Design review of the part shown in the three views and the two pictorial views. Dimensions are in mm from the part's minimum x, y and z. Coordinates: 2 decimals unless noted, no trailing zeros. Loops run counter-clockwise (first coordinate to the right, second up) from the corner with the lowest first, then second, coordinate; pieces in that order, holes last. Notation, with made-up numbers: (16, 66.5) -> (74, 66.5) arc R11 cw to (74, 80.5) -> close; hole circle Ø7 at (2.5, 72.25). An arc over 180 degrees is marked (long way). One line per item, written item: value. Start each with the question number.
1. Insertion check: pin 1 (3 mm diameter, centred on x = 2, z = 53, fed in from -Y); pin 2 (1 mm diameter, centred on y = 44, z = 12, fed in from -X); pin 3 (1.5 mm diameter, centred on x = 3, y = 40, fed in from -Z); pin 4 (2.5 mm diameter, centred on x = 3, y = 39, fed in from +Z). Each pin has a flat end and moves straight along its axis. Give the tip position at first contact, or say it passes through.
2. Add section D-D on y = 53. Write out the cut boundary in (x, z), plus the area to 3 significant figures.
3. Add section C-C on x = 2.2. Write out the cut boundary in (y, z).
4. Draft analysis for pull direction Z (two halves, no side actions). For the marked faces 1, 2 and 3, state which applies: pulls with the +Z half, pulls with the -Z half, needs draft (parallel to the pull), parting line crosses it, or undercut.
5. For probe 1 along Y at (x, z) = (4.8, 30.5) (1 decimal); probe 2 along Z at (x, y) = (2.7, 27.5) (1 decimal); probe 3 along Y at (x, z) = (4.3, 32), list the stretches that pass through material, from the lowest coordinate up.
6. Add section B-B on z = 30. Write out the cut boundary in (x, y), plus the area to 3 significant figures.
7. Add section A-A on y = 30. Write out the cut boundary in (x, z).
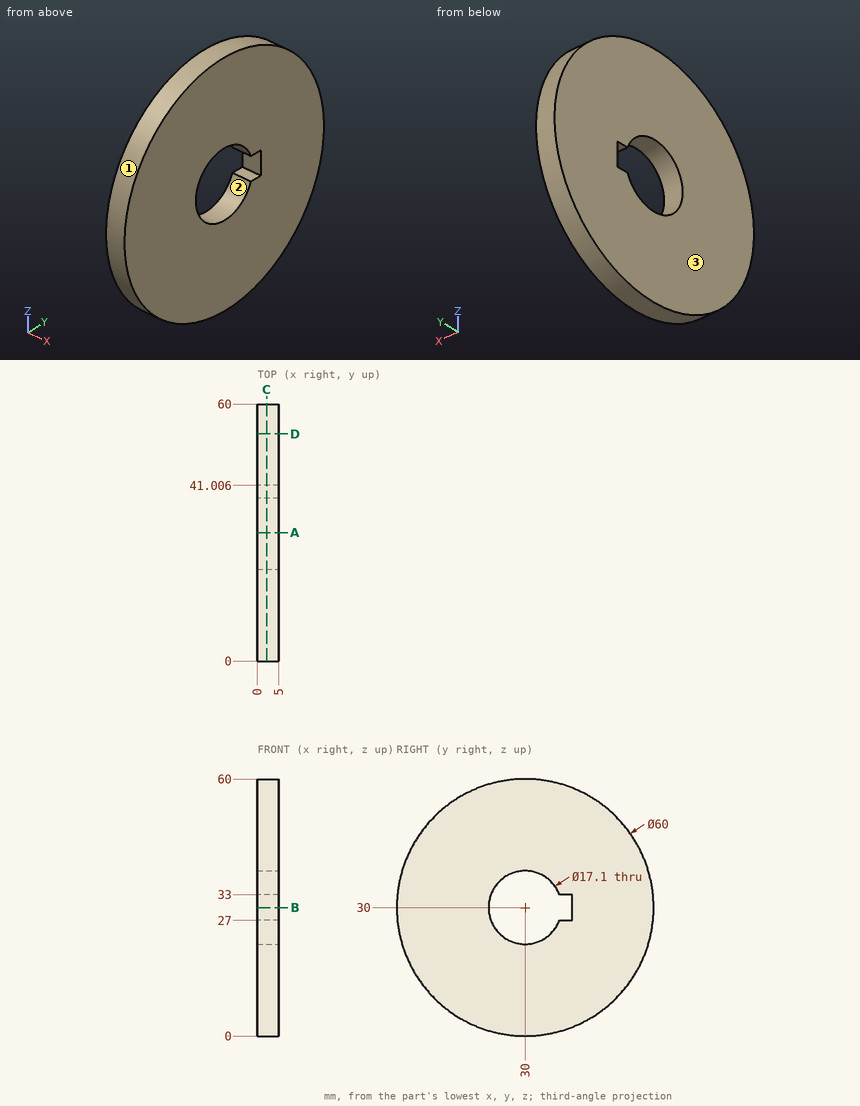
Worked answers:
1. pin 1: stops at y = 9.08
1. pin 2: stops at x = 0
1. pin 3: stops at z = 1.46
1. pin 4: stops at z = 58.98
2. outline: (0, 10.74) -> (5, 10.74) -> (5, 49.26) -> (0, 49.26) -> close
2. area: 193 mm²
3. outline: circle Ø60 at (30, 30); hole (38.01, 27) -> (41.01, 27) -> (41.01, 33) -> (38.01, 33) arc R8.55 ccw (long way) to start
4. face 1: parting line crosses it
4. face 2: undercut
4. face 3: needs draft
5. probe 1: y = 0 to 21.5, 41 to 60
5. probe 2: z = 0.1 to 21.8, 38.2 to 59.9
5. probe 3: y = 0.07 to 21.69, 41.01 to 59.93
6. outline: (0, 0) -> (5, 0) -> (5, 21.45) -> (0, 21.45) -> close; (0, 41.01) -> (5, 41.01) -> (5, 60) -> (0, 60) -> close
6. area: 202 mm²
7. outline: (0, 0) -> (5, 0) -> (5, 21.45) -> (0, 21.45) -> close; (0, 38.55) -> (5, 38.55) -> (5, 60) -> (0, 60) -> close
